```python
from build123d import *

# Parameters (mm, degrees)
PAD_DEPTH       = 0.8
SKETCH001_W     = 16
SKETCH001_H     = 8
POCKET_DEPTH    = 0.801
SKETCH002_R     = 1.5
POCKET001_DEPTH = 0.801
SKETCH003_R     = 2
POCKET002_DEPTH = 0.801


with BuildPart() as part:
    # Sketch → Pad (new body)
    with BuildSketch(Plane.XY):
        with BuildLine():
            ThreePointArc((4, 45), (1.171573, 43.828427), (0, 41))
            Line((0, 4), (0, 41))
            ThreePointArc((0, 4), (1.171573, 1.171573), (4, 0))
            Line((76, 0), (4, 0))
            ThreePointArc((76, 0), (78.828427, 1.171573), (80, 4))
            Line((80, 41), (80, 4))
            ThreePointArc((80, 41), (78.828427, 43.828427), (76, 45))
            Line((4, 45), (76, 45))
        make_face()
    extrude(amount=PAD_DEPTH)

    # Sketch001 (on Face10 of Pad) → Pocket (cut, through all)
    with BuildSketch(Plane.XY.offset(0.8)):
        with Locations((40, 22.5)):
            Rectangle(SKETCH001_W, SKETCH001_H)
    extrude(amount=-POCKET_DEPTH, mode=Mode.SUBTRACT)

    # Sketch002 (on Face5 of Pocket) → Pocket001 (cut, through all)
    with BuildSketch(Plane.XY.offset(0.8)):
        with Locations((55, 22.5)):
            Circle(SKETCH002_R)
        with Locations((25, 22.5)):
            Circle(SKETCH002_R)
    extrude(amount=-POCKET001_DEPTH, mode=Mode.SUBTRACT)

    # Sketch003 (on Face5 of Pocket001) → Pocket002 (cut, through all)
    with BuildSketch(Plane.XY.offset(0.8)):
        with Locations((6, 39)):
            Circle(SKETCH003_R)
        with Locations((74, 39)):
            Circle(SKETCH003_R)
        with Locations((74, 6)):
            Circle(SKETCH003_R)
        with Locations((6, 6)):
            Circle(SKETCH003_R)
    extrude(amount=-POCKET002_DEPTH, mode=Mode.SUBTRACT)


solid = part.part
```
Build history of the part. All positions in model axes, mm. Round coordinates to 2 decimals unless told otherwise and drop trailing zeros. Loops run counter-clockwise (first coordinate to the right, second up) from the corner with the lowest first, then second, coordinate; pieces in that order, holes last.
Item 1: Saw through at D-D (y = 22.5). List the corners of the cut face in (x, z), then the cut area to 3 significant figures.
Item 2: Two-plate mould, pull along X, no slides. Class faces 1 (the face through (23.89, 23.51, 0.41)), 2 (the face through (39, 18, 0.8)), 3 (the face through (78.859, 43.797, 0.394)): released by +X, released by -X, zero draft, split by the parting line, or undercut.
Item 3: Saw through at C-C (x = 55). List the corners of the cut face in (y, z), then the cut area to 3 significant figures.
Item 4: Saw through at A-A (y = 6). List the corners of the cut face in (x, z).
Item 5: Drill centre lines: line 1 along Y through (x, z) = (74, 0.25); line 2 along Y through (x, z) = (38.5, 0.65); line 3 along Y through (x, z) = (55, 0.6). Where is each one in solid material? Low to high.
Item 6: Saw through at B-B (z = 0.5). List the corners of the cut face in (x, y).
Worked answers:
1. outline: (0, 0) - (23.5, 0) - (23.5, 0.8) - (0, 0.8) - close; (26.5, 0) - (32, 0) - (32, 0.8) - (26.5, 0.8) - close; (48, 0) - (53.5, 0) - (53.5, 0.8) - (48, 0.8) - close; (56.5, 0) - (80, 0) - (80, 0.8) - (56.5, 0.8) - close
1. area: 46.4 mm2
2. face 1: undercut
2. face 2: zero draft
2. face 3: released by +X
3. outline: (0, 0) - (21, 0) - (21, 0.8) - (0, 0.8) - close; (24, 0) - (45, 0) - (45, 0.8) - (24, 0.8) - close
3. area: 33.6 mm2
4. outline: (0, 0) - (4, 0) - (4, 0.8) - (0, 0.8) - close; (8, 0) - (72, 0) - (72, 0.8) - (8, 0.8) - close; (76, 0) - (80, 0) - (80, 0.8) - (76, 0.8) - close
5. line 1: y = 0 to 4, 8 to 37, 41 to 45
5. line 2: y = 0 to 18.5, 26.5 to 45
5. line 3: y = 0 to 21, 24 to 45
6. outline: (0, 4) arc R4 ccw to (4, 0) - (76, 0) arc R4 ccw to (80, 4) - (80, 41) arc R4 ccw to (76, 45) - (4, 45) arc R4 ccw to (0, 41) - close; hole circle Ø4 at (6, 6); hole circle Ø4 at (6, 39); hole circle Ø3 at (25, 22.5); hole (32, 18.5) - (48, 18.5) - (48, 26.5) - (32, 26.5) - close; hole circle Ø3 at (55, 22.5); hole circle Ø4 at (74, 6); hole circle Ø4 at (74, 39)
